Answer from the drawing. Dimensions are ordinates in mm from the lowest x, y and z of the part. A direction names the side the tool comes from. Coordinates: 2 decimals unless noted, no trailing zeros. Write each loop counter-clockwise with the first axis right and the second up, starting at its lowest first coordinate (ties: lowest second). Pieces come first, ordered by that corner, then holes.
(1) For a pull along Z with two mould halves and no side action, classify the marked faces 1, 2 and 3 as +Z half, -Z half, draft (parallel to the pull), parting line (faces both ways), or undercut.
(2) The part is cut by section D-D on x = 22.5. Determine the outline of the cut face in (y, z), plus the area to 3 significant figures.
(3) Straight lines are drawn through the part: line 1 (Z direction, x = 2.5, y = 1.4); line 2 (Y direction, x = 16, z = 2.75); line 3 (Z direction, x = 9.75, y = 4.25). For each, find the intervals that lie inside material, in ascending order.
(4) The part is cut by section C-C on z = 9. Determine the outline of the cut face in (x, y), plus the area to 3 significant figures.
(5) Given P1, Ø12.5, axis at x = 14, z = 17.5, coming from the +Y side; P2, Ø2, axis at x = 14, y = 5, coming from the -Z side; P3, Ø3, axis at x = 22.5, z = 2.5, coming from the +Y side; P4, Ø2, axis at x = 2.5, z = 2.5, coming from the +Y side, each flat-ended and moving along its own axis, determine where each tip first touches the part or whether it passes through.
(6) The part is cut by section A-A on y = 2. Determine the outline of the cut face in (x, z).
(7) Which of the six approach directions +Z, -Z, +X, -X, +Y, -Y give full straight-line access (tool end or side, diameter ignored) to the marked faces 4, 5 and 6?
(8) The part is cut by section B-B on z = 2.5. Determine the outline of the cut face in (x, y).
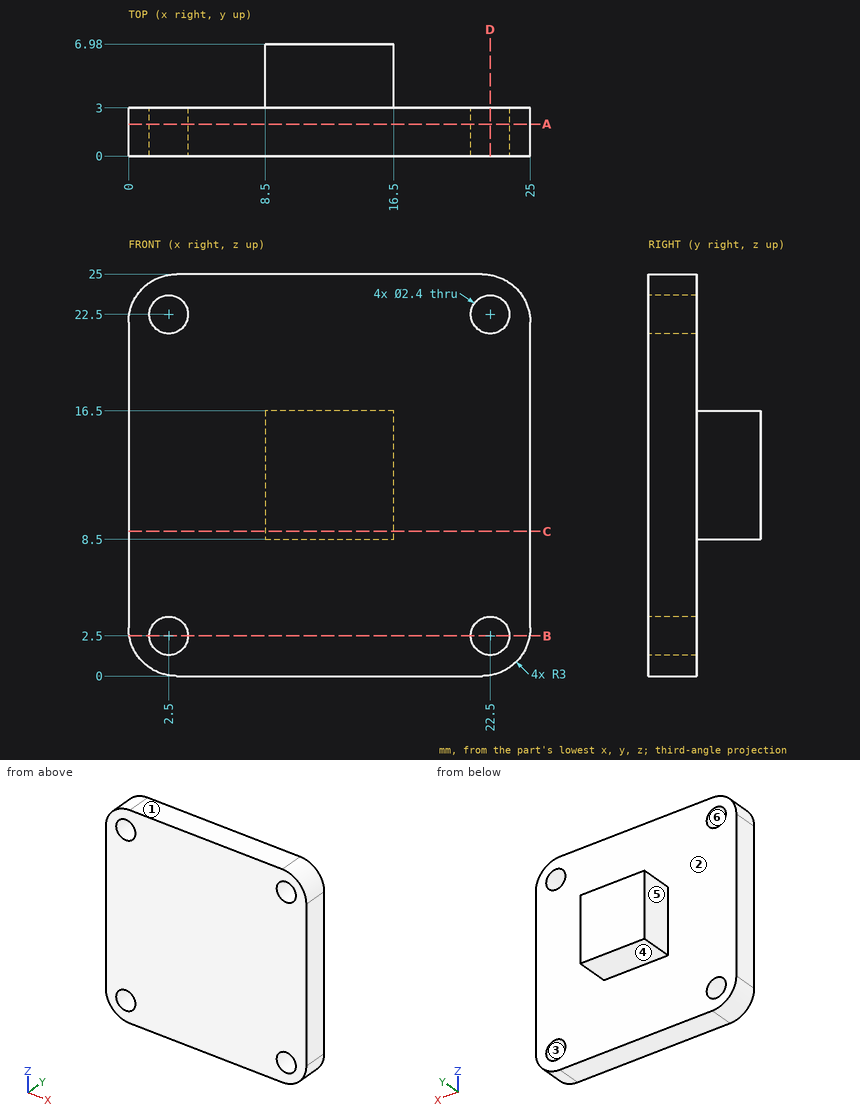
Model answer:
1. face 1: +Z half
1. face 2: draft
1. face 3: undercut
2. outline: (0, 0.04) - (3, 0.04) - (3, 1.3) - (0, 1.3) - close; (0, 3.7) - (3, 3.7) - (3, 21.3) - (0, 21.3) - close; (0, 23.7) - (3, 23.7) - (3, 24.96) - (0, 24.96) - close
2. area: 60.3 mm2
3. line 1: z = 0.04 to 1.3, 3.7 to 21.3, 23.7 to 24.96
3. line 2: y = 0 to 3
3. line 3: z = 8.5 to 16.5
4. outline: (0, 0) - (25, 0) - (25, 3) - (16.5, 3) - (16.5, 6.98) - (8.5, 6.98) - (8.5, 3) - (0, 3) - close
4. area: 107 mm2
5. P1: stops at y = 6.98
5. P2: stops at z = 8.5
5. P3: stops at y = 3
5. P4: passes through
6. outline: (0, 3) arc R3 ccw to (3, 0) - (22, 0) arc R3 ccw to (25, 3) - (25, 22) arc R3 ccw to (22, 25) - (3, 25) arc R3 ccw to (0, 22) - close; hole circle Ø2.4 at (2.5, 2.5); hole circle Ø2.4 at (2.5, 22.5); hole circle Ø2.4 at (22.5, 2.5); hole circle Ø2.4 at (22.5, 22.5)
7. face 4: -Z, +X, -X, +Y
7. face 5: +Z, -Z, -X, +Y
7. face 6: +Y, -Y
8. outline: (0.04, 0) - (1.3, 0) - (1.3, 3) - (0.04, 3) - close; (3.7, 0) - (21.3, 0) - (21.3, 3) - (3.7, 3) - close; (23.7, 0) - (24.96, 0) - (24.96, 3) - (23.7, 3) - close
